from build123d import *

# Parameters (mm, degrees)
F1_DEPTH = 5
F0_W     = 41.110674
F0_H     = 23.991064
F2_DEPTH = 25
F3_DEPTH = 25


with BuildPart() as f1:
    # F0 (on Top) → F1 (new body)
    with BuildSketch(Plane.XY):
        Polygon((96.131777, 26.425483), (-93.868223, 26.425483), (-93.868223, 11.705574), (-74.966818, 11.705574), (-74.966818, -11.828702), (-93.868223, -11.828702), (-93.868223, -14.370874), (-93.868223, -26.574517), (96.131777, -26.574517), (96.131777, -13.606817), (55.021103, -13.606817), (55.021103, 10.384247), (96.131777, 10.384247), align=None)
    extrude(amount=F1_DEPTH)

    # F0 (on Top) → F2 (cut)
    with BuildSketch(Plane.XY):
        Polygon((96.131777, 26.425483), (-93.868223, 26.425483), (-93.868223, 11.705574), (-74.966818, 11.705574), (-74.966818, -11.828702), (-93.868223, -11.828702), (-93.868223, -14.370874), (-93.868223, -26.574517), (96.131777, -26.574517), (96.131777, -13.606817), (55.021103, -13.606817), (55.021103, 10.384247), (96.131777, 10.384247), align=None)
        Polygon((-74.966818, 11.705574), (-93.868223, 11.705574), (-93.868223, -0.074517), (-93.868223, -11.828702), (-74.966818, -11.828702), align=None)
        with Locations((75.57644, -1.611285)):
            Rectangle(F0_W, F0_H)
    extrude(amount=-F2_DEPTH, mode=Mode.SUBTRACT)

    # F0 (on Top) → F3 (cut)
    with BuildSketch(Plane.XY):
        Polygon((96.131777, 26.425483), (-93.868223, 26.425483), (-93.868223, 11.705574), (-74.966818, 11.705574), (-74.966818, -11.828702), (-93.868223, -11.828702), (-93.868223, -14.370874), (-93.868223, -26.574517), (96.131777, -26.574517), (96.131777, -13.606817), (55.021103, -13.606817), (55.021103, 10.384247), (96.131777, 10.384247), align=None)
        Polygon((-74.966818, 11.705574), (-93.868223, 11.705574), (-93.868223, -0.074517), (-93.868223, -11.828702), (-74.966818, -11.828702), align=None)
        with Locations((75.57644, -1.611285)):
            Rectangle(F0_W, F0_H)
    extrude(amount=-F3_DEPTH, mode=Mode.SUBTRACT)


solid = f1.part
The model under review builds one solid part; all positions refer to its coordinate system, in mm. A direction names the side the tool comes from. Give positions to 0.01 mm unless a question says otherwise; leave off trailing zeros. Order: outer loops, then holes, each group sorted by start corner. A loop starts at its lowest first (then second) coordinate and runs counter-clockwise, first axis right, second up. Notation, with made-up numbers: M -29.5,-12.5 L 20.5,-12.5 A15 ccw 20.5,-8.5 Z; hole C 82.5,-5 d10. An arc over 180 degrees is marked long. Answer in a Markdown table with one row per item. Add a question column.
1. Add section B-B on y = 6. State the section outline as (x, z) points, plus the area to 3 significant figures.
2. To check wall thickness, follow line 1 along Y through (x, z) = (59, 4.65); line 2 along X through (y, z) = (-9.5, 3.2). State the ranges of each line that lie inside material, in increasing order.
3. Add section A-A on z = 3.75. State the section outline as (x, y) points.
4. Machinability: for faces 1 (the flat face through (0, 0, 0)), 2 (the flat face through (76, -13.607, 2)), 3 (the flat face through (-85, 11.706, 2)), which of the approach directions +Z, -Z, +X, -X, +Y, -Y give a long, thin tool a straight path to every point of the face, cutting with its end or side? Answer none if there is none.
5. For pin 1 Ø3 at (y, z) = (2, 2) entering from -X, flat-tipped, find the tip position at first contact; note if it passes through.
6. Mouldability with a two-part tool opening along Y and no side actions: class faces 4 (the flat face through (0, -26.575, 2)), 5 (the flat face through (75, 10.384, 2)), 6 (the flat face through (-74.967, 0, 2)), 7 (the flat face through (-93.868, 19, 2)) as released by +Y, released by -Y, zero draft, split by the parting line, or undercut.
The answers:
| question | item | result |
|---|---|---|
| 1 | outline | M -74.97,0 L 55.02,0 L 55.02,5 L -74.97,5 Z |
| 1 | area | 650 mm2 |
| 2 | line 1 | -26.57 to -13.61, 10.38 to 26.43 |
| 2 | line 2 | -74.97 to 55.02 |
| 3 | outline | M -93.87,-26.57 L 96.13,-26.57 L 96.13,-13.61 L 55.02,-13.61 L 55.02,10.38 L 96.13,10.38 L 96.13,26.43 L -93.87,26.43 L -93.87,11.71 L -74.97,11.71 L -74.97,-11.83 L -93.87,-11.83 Z |
| 4 | face 1 | -Z, +X, -X, +Y, -Y |
| 4 | face 2 | +Z, -Z, +X |
| 4 | face 3 | +Z, -Z, -X |
| 5 | pin 1 | x = -74.97 |
| 6 | face 4 | released by -Y |
| 6 | face 5 | undercut |
| 6 | face 6 | undercut |
| 6 | face 7 | zero draft |
